Part print with two shaded views. Sizes in mm from the minimum x, y, z corner. A direction names the side the tool comes from. Coordinates: 2 decimals unless noted, no trailing zeros. Order: outer loops, then holes, each group sorted by start corner. A loop starts at its lowest first (then second) coordinate and runs counter-clockwise, first axis right, second up. Notation, with made-up numbers: M 27,66 L 39,66 A31 ccw 39,103 Z; hole C 73.5,2.25 d4. An arc over 180 degrees is marked long. Answer in a Markdown table with one row per item. Add a question column.
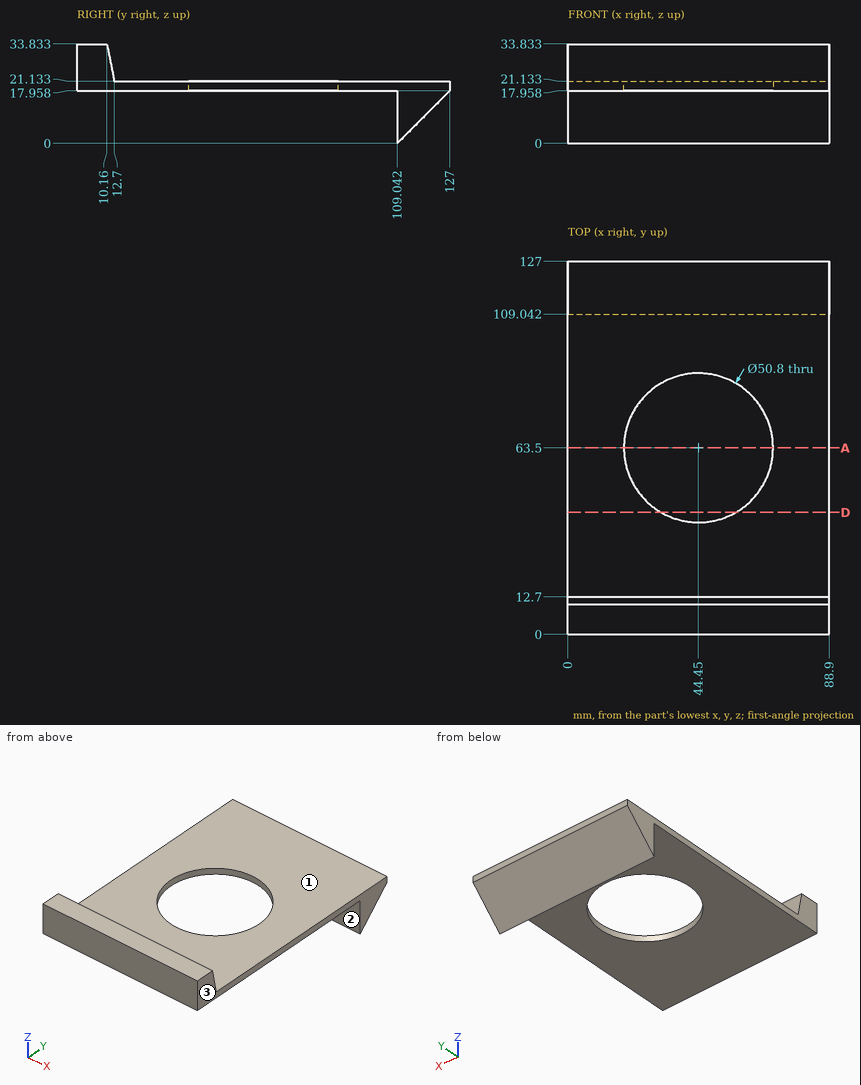
(1) Slice it at D-D (y = 41.5). List the corners of the cut face in (x, z) (1 decimal), and give its area (3 significant figures).
(2) Wall check: line 1 (Y direction, x = 44.45, z = 20.3); line 2 (X direction, y = 52, z = 19.5); line 3 (Z direction, x = 6, y = 69.5). Give the ranges that are in metal, low to high.
(3) Slice it at A-A (y = 63.5). List the corners of the cut face in (x, z), and give its area (3 significant figures).
(4) Drop flat-ended pins along their axis: P1, Ø6, axis at x = 42.5, y = 21.5, coming from the -Z side; P2, Ø5, axis at x = 33, y = 31, coming from the +Z side; P3, Ø12, axis at x = 62.5, z = 21.5, coming from the -Y side; P4, Ø14.5, axis at x = 45, z = 7.5, coming from the -Y side. Give the stop position or say it passes through.
(5) 3-axis set-ups, long thin cutter, end or side, ignore diameter. For the marked faces 1, 2 and 3: which of +Z, -Z, +X, -X, +Y, -Y reach the whole face in a straight line?
Computed:
| question | item | result |
|---|---|---|
| 1 | outline | M 0,18 L 31.8,18 L 31.8,21.1 L 0,21.1 Z; M 57.1,18 L 88.9,18 L 88.9,21.1 L 57.1,21.1 Z |
| 1 | area | 202 mm^2 |
| 2 | line 1 | y = 0 to 38.1, 88.9 to 127 |
| 2 | line 2 | x = 0 to 21.8, 67.1 to 88.9 |
| 2 | line 3 | z = 17.96 to 21.13 |
| 3 | outline | M 0,17.96 L 19.05,17.96 L 19.05,21.13 L 0,21.13 Z; M 69.85,17.96 L 88.9,17.96 L 88.9,21.13 L 69.85,21.13 Z |
| 3 | area | 121 mm^2 |
| 4 | P1 | stops at z = 17.96 |
| 4 | P2 | stops at z = 21.13 |
| 4 | P3 | stops at y = 0 |
| 4 | P4 | stops at y = 109.04 |
| 5 | face 1 | +Z, +X, -X, +Y |
| 5 | face 2 | -Z, +X, -X, -Y |
| 5 | face 3 | +Z, -Z, +X, +Y, -Y |
